The drawing under review shows one solid part. Ordinate dimensions are in mm from its lowest x, y, z. Coordinates: 2 decimals unless noted, no trailing zeros. Write each loop counter-clockwise with the first axis right and the second up, starting at its lowest first coordinate (ties: lowest second). Pieces come first, ordered by that corner, then holes. Notation, with made-up numbers: (-11, 83) - (10, 83) arc R15 ccw to (10, 92) - close; hole circle Ø5 at (-4, 55). An arc over 180 degrees is marked (long way). Use a Markdown table: item, result.
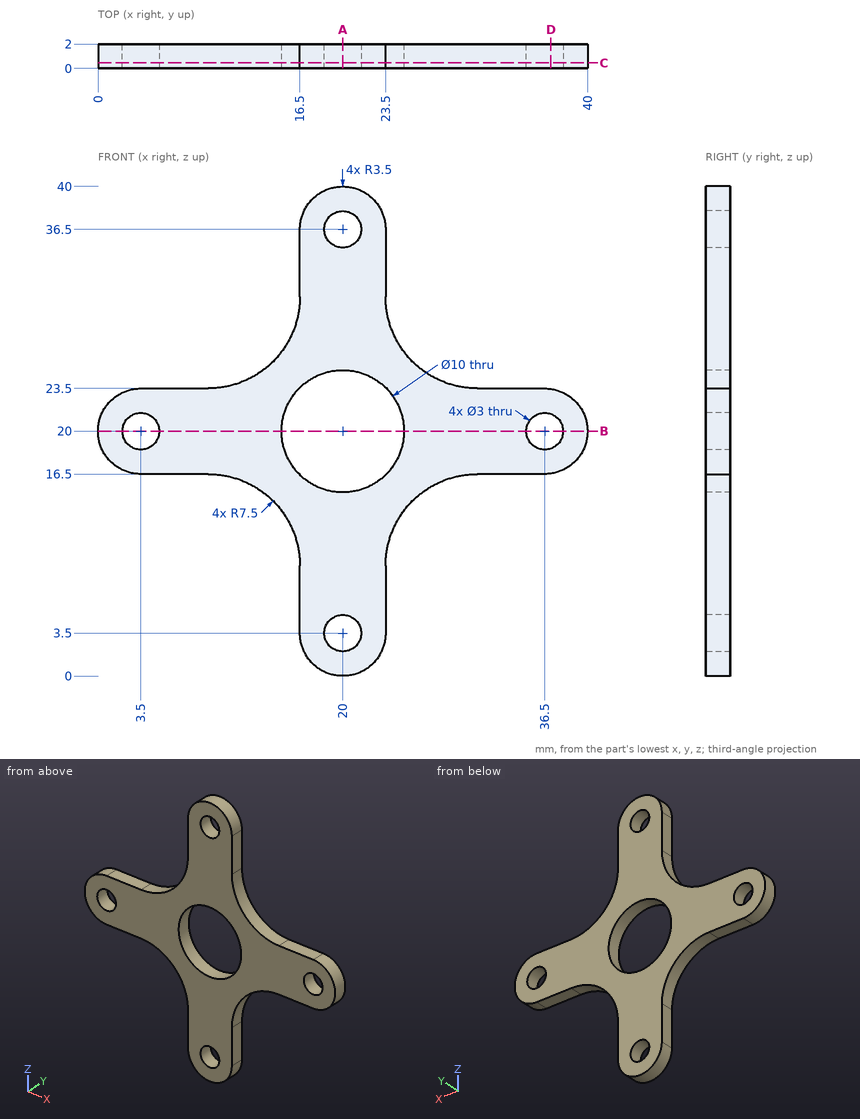
(1) Take a section at C-C on y = 0.45. Write out the cut boundary in (x, z).
Determined:
| item | result |
|---|---|
| outline | (3.5, 16.5) - (9, 16.5) arc R7.5 cw to (16.5, 9) - (16.5, 3.5) arc R3.5 ccw to (23.5, 3.5) - (23.5, 9) arc R7.5 cw to (31, 16.5) - (36.5, 16.5) arc R3.5 ccw to (36.5, 23.5) - (31, 23.5) arc R7.5 cw to (23.5, 31) - (23.5, 36.5) arc R3.5 ccw to (16.5, 36.5) - (16.5, 31) arc R7.5 cw to (9, 23.5) - (3.5, 23.5) arc R3.5 ccw to start; hole circle Ø3 at (3.5, 20); hole circle Ø10 at (20, 20); hole circle Ø3 at (20, 3.5); hole circle Ø3 at (20, 36.5); hole circle Ø3 at (36.5, 20) |
(2) For L1, parallel to Z at x = 20, y = 1.1; L2, parallel to Z at x = 3.5, y = 1.15; L3, parallel to X at y = 1.75, z = 26.5, list the stretches that pass through material, from the lowest coordinate up. Write a range as from..to.
Determined:
| item | result |
|---|---|
| L1 | 0..2, 5..15, 25..35, 38..40 |
| L2 | 16.5..18.5, 21.5..23.5 |
| L3 | 15..25 |
(3) Take a section at D-D on x = 37. Write out the cut boundary in (y, z), and give its area (3 significant figures).
Determined:
| item | result |
|---|---|
| outline | (0, 16.54) - (2, 16.54) - (2, 18.59) - (0, 18.59) - close; (0, 21.41) - (2, 21.41) - (2, 23.46) - (0, 23.46) - close |
| area | 8.20 mm2 |
(4) For pin 1 (1 mm diameter, centred on x = 35, y = 1.5, fed in from -Z); pin 2 (4 mm diameter, centred on x = 20, z = 3.5, fed in from -Y); pin 3 (1 mm diameter, centred on x = 32.5, y = 0.5, fed in from +Z); pin 4 (0.6 mm diameter, centred on y = 0.5, z = 6, fed in from -X), all flat-tipped, find the tip position at first contact; note any pin that passes through.
Determined:
| item | result |
|---|---|
| pin 1 | z = 16.5 |
| pin 2 | y = 0 |
| pin 3 | z = 23.5 |
| pin 4 | x = 16.5 |
(5) Take a section at B-B on z = 20. Write out the cut boundary in (x, y), and give its area (3 significant figures).
Determined:
| item | result |
|---|---|
| outline | (0, 0) - (2, 0) - (2, 2) - (0, 2) - close; (5, 0) - (15, 0) - (15, 2) - (5, 2) - close; (25, 0) - (35, 0) - (35, 2) - (25, 2) - close; (38, 0) - (40, 0) - (40, 2) - (38, 2) - close |
| area | 48.0 mm2 |
(6) Take a section at A-A on x = 20. Write out the cut boundary in (y, z).
Determined:
| item | result |
|---|---|
| outline | (0, 0) - (2, 0) - (2, 2) - (0, 2) - close; (0, 5) - (2, 5) - (2, 15) - (0, 15) - close; (0, 25) - (2, 25) - (2, 35) - (0, 35) - close; (0, 38) - (2, 38) - (2, 40) - (0, 40) - close |
